Could you check a few things on this drawing? It's one solid part, dimensions in mm from its lowest x, y, z. A direction names the side the tool comes from. Give positions to 0.01 mm unless a question says otherwise; leave off trailing zeros. Loops run counter-clockwise (first coordinate to the right, second up) from the corner with the lowest first, then second, coordinate; pieces in that order, holes last. Notation, with made-up numbers: (12, -8) - (65, -8) arc R32 cw to (65, 28) - close; hole circle Ø2 at (48.25, -18). An arc over 180 degrees is marked (long way). Use CSV: the item, a comma, the result in double quotes.
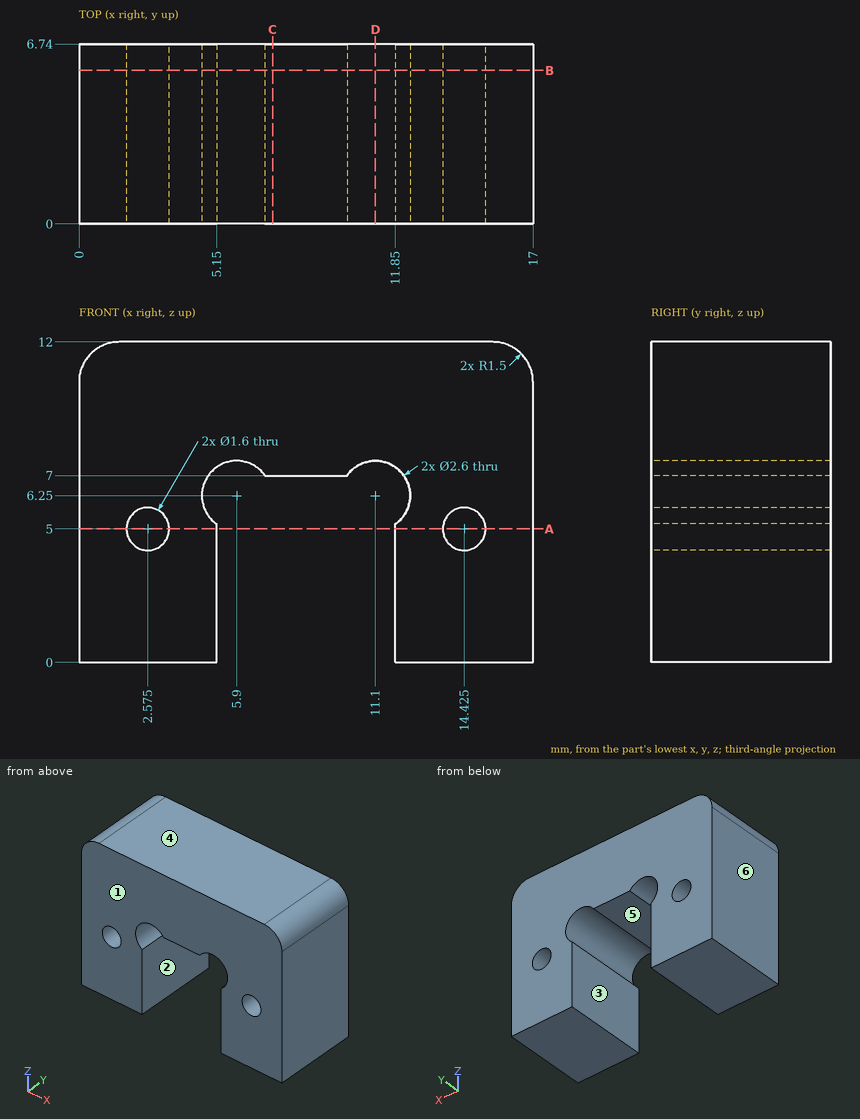
1) Which directions (+Z, -Z, +X, -X, +Y, -Y) give clear straight access to the entire face, cutting with the end or side of a thin tool? Please do the marked faces 1 and 2.
Answer below:
face 1,"+Z, -Z, +X, -X, -Y"
face 2,"-Z, +Y, -Y"
2) I'm going to push flat-ended pins straight in: P1, Ø4, axis at x = 5.9, z = 6.25, coming from the +Y side; P2, Ø1.5, axis at x = 9, y = 4.5, coming from the -Z side. Where does each tip first touch, or does it pass through?
Answer below:
P1,"stops at y = 6.74"
P2,"stops at z = 7"
3) I need wall thicknesses on line 1 along X through (y, z) = (1, 4.5); line 2 along X through (y, z) = (1.25, 0.75). Which ranges of each line are inside material? Lowest first, please.
Answer below:
line 1,"x = 0 to 1.95, 3.2 to 5.15, 11.85 to 13.8, 15.05 to 17"
line 2,"x = 0 to 5.15, 11.85 to 17"
4) Suppose I cut it at D-D (x = 11.1). Please give me the cut outline in (y, z).
Answer below:
outline,"(0, 7.55) - (6.74, 7.55) - (6.74, 12) - (0, 12) - close"
5) We'd pull the mould along X, two halves only. Please class the marked faces 3, 4, 5 and 6: +X half, -X half, draft (parallel to the pull), parting line (faces both ways), or undercut.
Answer below:
face 3,"undercut"
face 4,"draft"
face 5,"undercut"
face 6,"-X half"
6) Suppose I cut it at C-C (x = 7.25). Please give me the cut outline in (y, z), plus the area to 3 significant figures.
Answer below:
outline,"(0, 7) - (6.74, 7) - (6.74, 12) - (0, 12) - close"
area,"33.7 mm2"
7) Suppose I cut it at B-B (y = 5.75). Please give me the cut outline in (x, z) (3 decimals).
Answer below:
outline,"(0, 0) - (5.15, 0) - (5.15, 5.188) arc R1.3 cw (long way) to (6.962, 7) - (10.038, 7) arc R1.3 cw (long way) to (11.85, 5.188) - (11.85, 0) - (17, 0) - (17, 10.5) arc R1.5 ccw to (15.5, 12) - (1.5, 12) arc R1.5 ccw to (0, 10.5) - close; hole circle Ø1.6 at (2.575, 5); hole circle Ø1.6 at (14.425, 5)"
8) Suppose I cut it at A-A (z = 5). Please give me the cut outline in (x, y) (3 decimals).
Answer below:
outline,"(0, 0) - (1.775, 0) - (1.775, 6.74) - (0, 6.74) - close; (3.375, 0) - (5.15, 0) - (5.15, 6.74) - (3.375, 6.74) - close; (11.85, 0) - (13.625, 0) - (13.625, 6.74) - (11.85, 6.74) - close; (15.225, 0) - (17, 0) - (17, 6.74) - (15.225, 6.74) - close"
